Check sheet for the drawn part. Datum: minimum x, y, z corner. Units: mm. Round coordinates to 2 decimals unless told otherwise and drop trailing zeros. Write each loop counter-clockwise with the first axis right and the second up, starting at its lowest first coordinate (ties: lowest second). Pieces come first, ordered by that corner, then holes. Notation, with made-up numbers: M -1.5,66.5 L 21.5,66.5 A12 ccw 21.5,84.5 Z; hole C 29.25,3 d8. An arc over 180 degrees is marked long. One line per item, written item: value. Start each with the question number.
1. Depth check by flat-ended pin: P1, Ø5.5, axis at x = 98.5, z = 82, coming from the +Y side (3 decimals). Enter the tip coordinate at first touch or a pass-through.
2. Section check A-A (y = 14). Record the boundary of the cut face in (x, z).
3. Scan lines: probe 1 along Z at (x, y) = (43.5, 12.75); probe 2 along Y at (x, z) = (99, 82) (3 decimals). Record each from-to range of solid material in increasing order. Write a range as [from, to].
4. Section check B-B (x = 70.5). Record the boundary of the cut face in (y, z) (3 decimals), and give its area (3 significant figures).
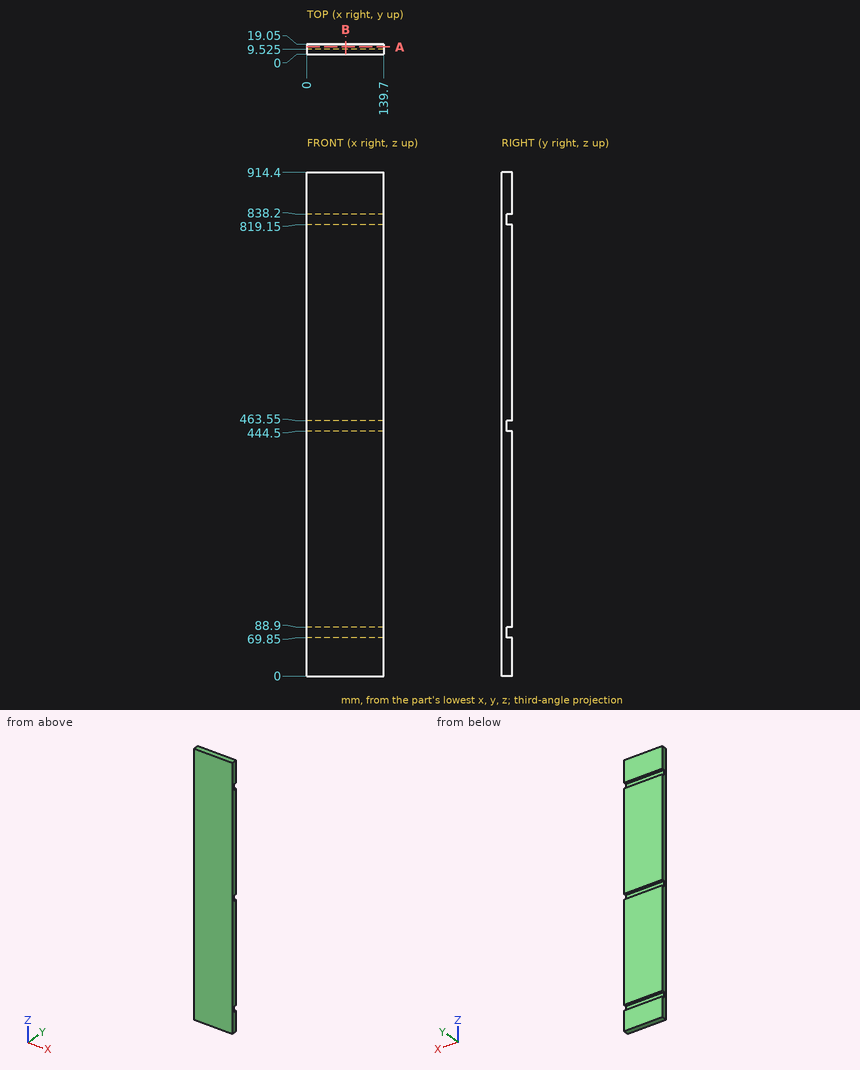
Result sheet:
1. P1: stops at y = 9.525
2. outline: M 0,0 L 139.7,0 L 139.7,69.85 L 0,69.85 Z; M 0,88.9 L 139.7,88.9 L 139.7,444.5 L 0,444.5 Z; M 0,463.55 L 139.7,463.55 L 139.7,819.15 L 0,819.15 Z; M 0,838.2 L 139.7,838.2 L 139.7,914.4 L 0,914.4 Z
3. probe 1: z = [0, 69.85], [88.9, 444.5], [463.55, 819.15], [838.2, 914.4]
3. probe 2: y = [0, 9.525]
4. outline: M 0,0 L 19.05,0 L 19.05,69.85 L 9.525,69.85 L 9.525,88.9 L 19.05,88.9 L 19.05,444.5 L 9.525,444.5 L 9.525,463.55 L 19.05,463.55 L 19.05,819.15 L 9.525,819.15 L 9.525,838.2 L 19.05,838.2 L 19.05,914.4 L 0,914.4 Z
4. area: 16,900 mm2
